Here's the drawing with two shaded views (mm, measured from the low corner). I have some questions. Give positions to 0.01 mm unless a question says otherwise; leave off trailing zeros. Loops run counter-clockwise (first coordinate to the right, second up) from the corner with the lowest first, then second, coordinate; pieces in that order, holes last. Notation, with made-up numbers: (41, 17) -> (45, 17) arc R21 ccw to (45, 32) -> close; hole circle Ø9 at (-21.5, -20.5). An arc over 180 degrees is marked (long way). Put each result on its own line as item: value.
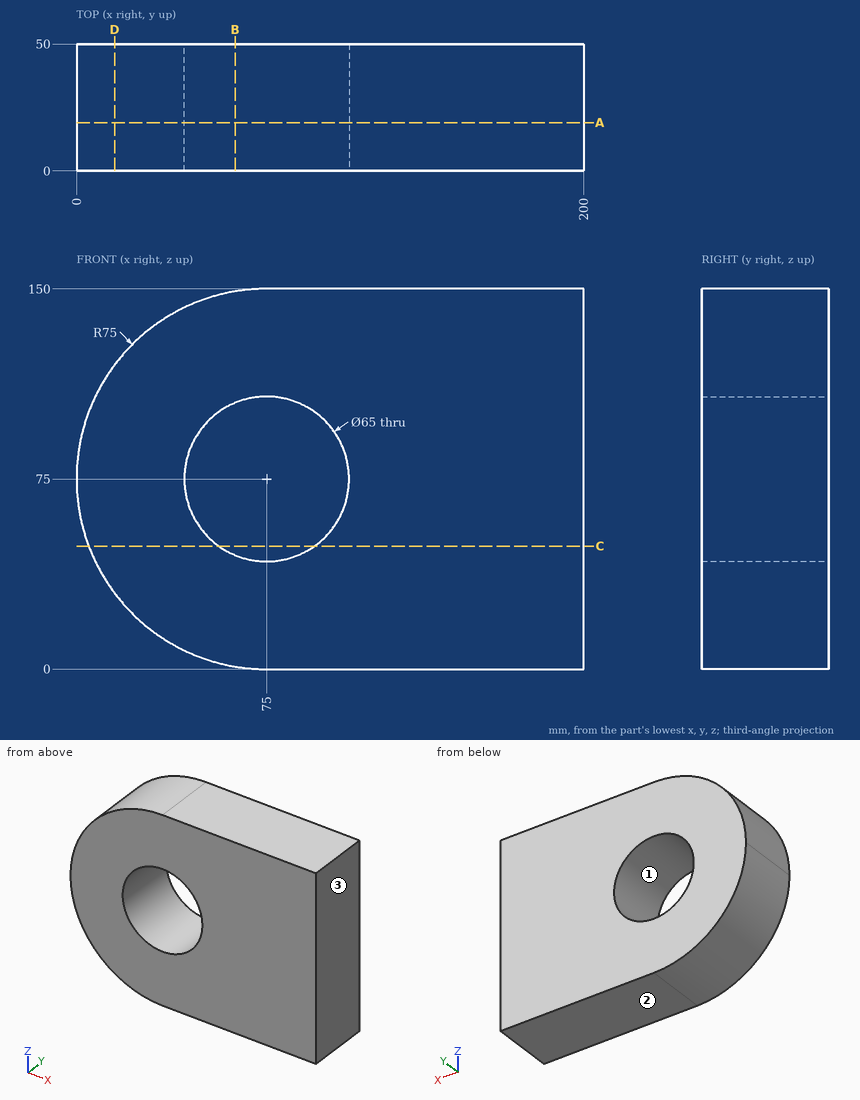
1. If we section it at D-D (x = 15): List the corners of the cut face in (y, z) for me.
Recorded:
outline: (0, 30) -> (50, 30) -> (50, 120) -> (0, 120) -> close
2. If we section it at A-A (y = 19): List the corners of the cut face in (x, z) for me, then the cut area to 3 significant figures.
Recorded:
outline: (0, 75) arc R75 ccw to (75, 0) -> (200, 0) -> (200, 150) -> (75, 150) arc R75 ccw to start; hole circle Ø65 at (75, 75)
area: 24,300 mm^2
3. If we section it at C-C (z = 48.5): List the corners of the cut face in (x, y) for me, then the cut area to 3 significant figures.
Recorded:
outline: (4.84, 0) -> (56.19, 0) -> (56.19, 50) -> (4.84, 50) -> close; (93.81, 0) -> (200, 0) -> (200, 50) -> (93.81, 50) -> close
area: 7,880 mm^2
4. I need wall thicknesses on line 1 (Z direction, x = 75, y = 36); line 2 (X direction, y = 38.5, z = 62); line 3 (X direction, y = 35, z = 59). Which ranges of each line are inside material? Lowest first, please.
Recorded:
line 1: z = 0 to 42.5, 107.5 to 150
line 2: x = 1.14 to 45.21, 104.79 to 200
line 3: x = 1.73 to 46.71, 103.29 to 200
5. If we section it at B-B (x = 62.5): List the corners of the cut face in (y, z) for me, then the cut area to 3 significant figures.
Recorded:
outline: (0, 1.05) -> (50, 1.05) -> (50, 45) -> (0, 45) -> close; (0, 105) -> (50, 105) -> (50, 148.95) -> (0, 148.95) -> close
area: 4,400 mm^2
6. Thinking about a two-plate mould opening in Z: for the marked faces 1, 2 and 3, which applies, pulls with the +Z half, pulls with the -Z half, needs draft (parallel to the pull), parting line crosses it, or undercut?
Recorded:
face 1: undercut
face 2: pulls with the -Z half
face 3: needs draft
7. I'm going to push flat-ended pins straight in: pin 1 (1 mm diameter, centred on y = 36, z = 115.5, fed in from -X); pin 2 (3 mm diameter, centred on y = 37, z = 62.5, fed in from -X); pin 3 (1 mm diameter, centred on y = 10, z = 42, fed in from -X). Where does each tip first touch, or does it pass through?
Recorded:
pin 1: stops at x = 11.56
pin 2: stops at x = 0.81
pin 3: stops at x = 7.41
